Geometry check sheet. Reference: drawing and pictorial views, mm from the part's lowest x, y, z. Coordinates: 2 decimals unless noted, no trailing zeros. Loops run counter-clockwise (first coordinate to the right, second up) from the corner with the lowest first, then second, coordinate; pieces in that order, holes last. Notation, with made-up numbers: (-39, 85) -> (-7, 85) arc R19 cw to (-7, 99) -> close; hole circle Ø3 at (-30, 12.25). An arc over 180 degrees is marked (long way). Use one line per item in the form item = value.
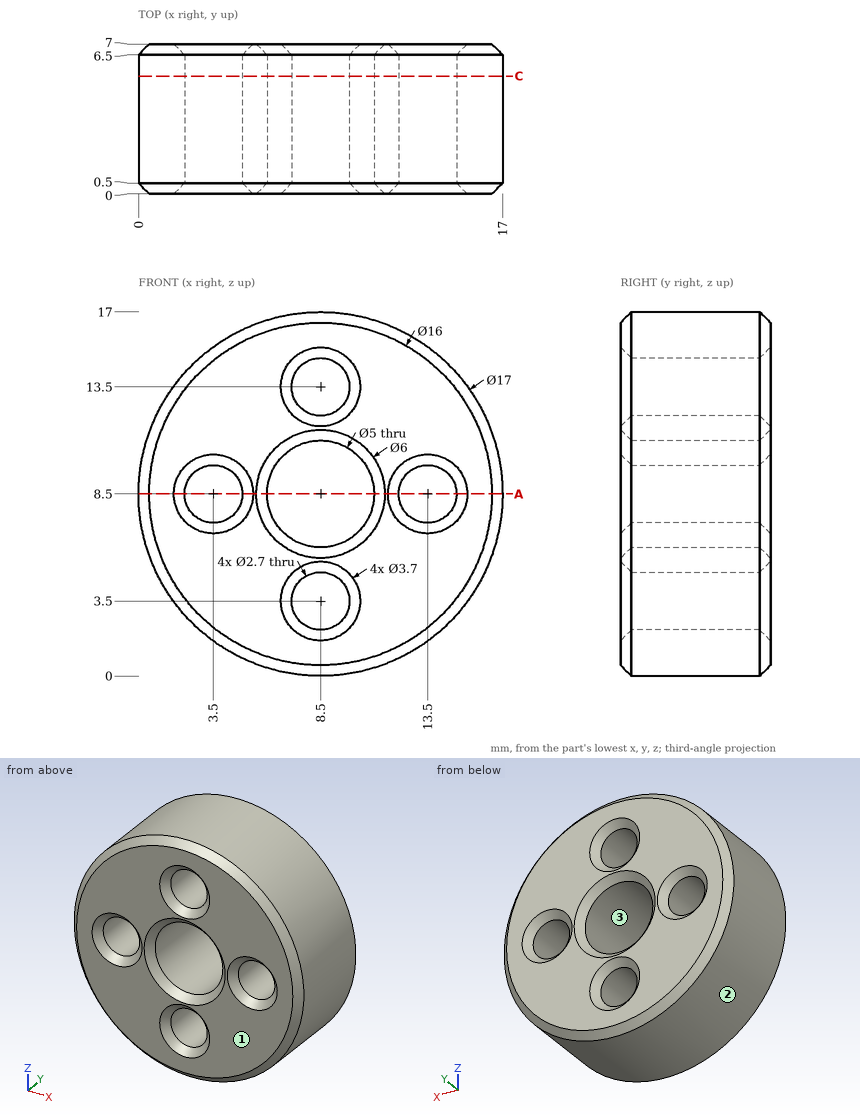
(1) Scan lines: line 1 along X through (y, z) = (3.55, 8.5); line 2 along X through (y, z) = (1.5, 7.75); line 3 along X through (y, z) = (2.75, 14.25). Record each from-to range of solid material in increasing order.
Established:
line_1 = 0 to 2.15, 4.85 to 6, 11 to 12.15, 14.85 to 17
line_2 = 0.03 to 2.38, 4.62 to 6.12, 10.88 to 12.38, 14.62 to 16.97
line_3 = 2.24 to 7.38, 9.62 to 14.76
(2) Section check C-C, the plane y = 5.5. Record the boundary of the cut face in (x, z), plus the area to 3 significant figures.
Established:
outline = circle Ø17 at (8.5, 8.5); hole circle Ø2.7 at (3.5, 8.5); hole circle Ø5 at (8.5, 8.5); hole circle Ø2.7 at (8.5, 3.5); hole circle Ø2.7 at (8.5, 13.5); hole circle Ø2.7 at (13.5, 8.5)
area = 184 mm²
(3) Mould release check, pull along X, two halves, no side actions. Record for the marked faces 1, 2 and 3: +X half, -X half, draft (parallel to the pull), parting line (faces both ways), or undercut.
Established:
face_1 = draft
face_2 = parting line
face_3 = undercut
(4) Section check A-A, the plane z = 8.5. Give the number of separate pieces and of enclosed holes in the cut face, plus the area to 3 significant figures.
Established:
separate_pieces = 4
enclosed_holes = 0
area = 44.2 mm²
(5) Go/stop test with flat-tipped pins: P1, Ø4, axis at x = 1.5, y = 3, coming from the -Z side; P2, Ø2, axis at y = 4, z = 4, coming from the +X side; P3, Ø3, axis at x = 8.5, z = 3.5, coming from the +Y side. Record where each tip stops, or that it passes through.
Established:
P1 = 1.63
P2 = 16.25
P3 = 6.65
